Input: part model. Units: mm. Frame: model coordinates. Face numbers are marked on the shaded views. A direction names the side the tool comes from. Round coordinates to 2 decimals unless told otherwise and drop trailing zeros. Order: outer loops, then holes, each group sorted by start corner. A loop starts at its lowest first (then second) coordinate and runs counter-clockwise, first axis right, second up.
Item 1: Cut plane C-C on x = 10.25. Output: boundary loops of the cut face in (y, z).
Item 2: Line query: L1, parallel to Y at x = -1.8, z = -0.05; L2, parallel to Y at x = 4, z = 0; L3, parallel to X at y = -0.45, z = 0.3. Output: solid intervals per line, ascending.
Item 3: Mould query, pull axis Y, two halves, no side actions, for the marked faces 5, 6 and 7. Classes: released by +Y, released by -Y, zero draft, split by the parting line, or undercut.
Item 4: Cut plane B-B on y = 0. Output: boundary loops of the cut face in (x, z).
Item 5: Cut plane D-D on x = 3. Output: boundary loops of the cut face in (y, z), then the cut area to 3 significant figures.
Item 6: Cut plane A-A on x = -1.8. Output: boundary loops of the cut face in (y, z), then the cut area to 3 significant figures.
Item 7: Reachability of the marked faces 1, 2, 3 and 4 from +Z, -Z, +X, -X, +Y, -Y: full face, straight path, thin tool, end or side. Return the list, or none.
```python
from build123d import *

# Parameters (mm, degrees)
CUT_EXTRUDE1_DEPTH      = 13.655828697
CUT_EXTRUDE1_DEPTH_BACK = 13.655828697
CUT_EXTRUDE2_DEPTH      = 13.597618823
CUT_EXTRUDE2_DEPTH_BACK = 13.597618823


with BuildPart() as part:
    # Sketch1 → Revolve1 (revolve)
    with BuildSketch(Plane.XY, mode=Mode.PRIVATE) as revolve1_sk:
        with BuildLine():
            Line((0, 0.7), (-1.203701126, 1.266660038))
            ThreePointArc((-1.203701126, 1.266660038), (-2.550060523, 1.182120642), (-3.2, 0))
            Line((-3.2, 0), (12.5, 0))
            Line((12.5, 0), (12.5, 0.7))
            Line((12.5, 0.7), (0, 0.7))
        make_face()
    revolve(revolve1_sk.sketch.rotate(Axis((0, 0, 0), (1, 0, 0)), 90), axis=Axis((0, 0, 0), (1, 0, 0)))

    # Sketch2 → Cut-Extrude1 (cut, two sides: drawn at the far end of the back side and taken through both)
    with BuildSketch(Plane(origin=(0, 0, 0), x_dir=(1, 0, 0), z_dir=(0, 1, 0)).offset(-CUT_EXTRUDE1_DEPTH_BACK)):
        with BuildLine():
            Line((-3.012435565, 0.7), (0, 0.7))
            Line((0, 0.7), (-1.203701126, 1.266660038))
            ThreePointArc((-1.203701126, 1.266660038), (-2.218547495, 1.335970806), (-3.012435565, 0.7))
        make_face()
        with BuildLine():
            Line((-3.012435565, -0.7), (0, -0.7))
            Line((0, -0.7), (-1.203701126, -1.266660038))
            ThreePointArc((-1.203701126, -1.266660038), (-2.218547495, -1.335970806), (-3.012435565, -0.7))
        make_face()
    extrude(amount=CUT_EXTRUDE1_DEPTH + CUT_EXTRUDE1_DEPTH_BACK, mode=Mode.SUBTRACT)

    # Sketch3 → Cut-Extrude2 (cut, two sides: drawn at the far end of the back side and taken through both)
    with BuildSketch(Plane.XY.offset(-CUT_EXTRUDE2_DEPTH_BACK)):
        with BuildLine():
            Line((-1.530011672, 0.645837675), (-0.32, 0.14))
            Line((-0.32, 0.14), (10, 0.14))
            Line((10, 0.14), (10, 0.7))
            Line((10, 0.7), (12.5, 0.7))
            Line((12.5, 0.7), (12.5, -0.14))
            Line((12.5, -0.14), (-0.32, -0.14))
            Line((-0.32, -0.14), (-1.530011672, -0.645837675))
            ThreePointArc((-1.530011672, -0.645837675), (-2.5, 0), (-1.530011672, 0.645837675))
        make_face()
    extrude(amount=CUT_EXTRUDE2_DEPTH + CUT_EXTRUDE2_DEPTH_BACK, mode=Mode.SUBTRACT)


solid = part.part
```
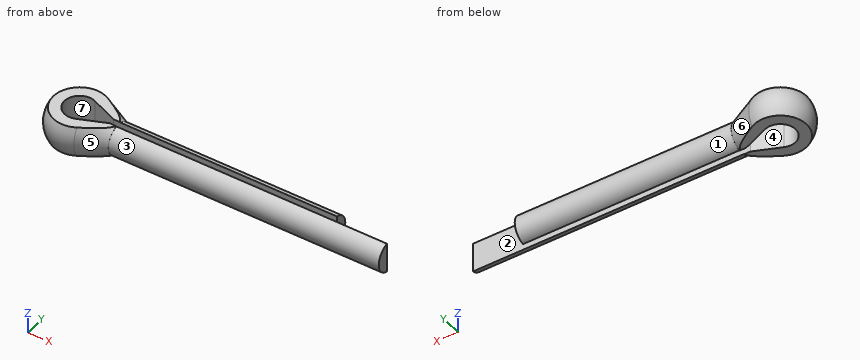
From the geometry:
1. outline: (-0.14, -0.69) - (-0.14, 0.69) arc R0.7 ccw to start
2. L1: y = -1.4 to -0.7, 0.7 to 1.4
2. L2: y = -0.7 to -0.14, 0.14 to 0.7
2. L3: x = -3.09 to -2.34, -1.06 to 12.5
3. face 5: released by -Y
3. face 6: released by +Y
3. face 7: undercut
4. outline: (-3.01, -0.7) - (-2.5, -0.7) - (-2.5, 0.7) - (-3.01, 0.7) arc R1.4 ccw to start
5. outline: (-0.14, -0.69) - (-0.14, 0.69) arc R0.7 ccw to start; (0.14, -0.69) arc R0.7 ccw to (0.14, 0.69) - close
5. area: 1.15 mm2
6. outline: (-1.21, -0.7) - (-0.7, -0.7) - (-0.7, 0.7) - (-1.21, 0.7) arc R1.4 ccw to start; (0.7, -0.7) - (1.21, -0.7) arc R1.4 ccw to (1.21, 0.7) - (0.7, 0.7) - close
6. area: 1.79 mm2
7. face 1: +X, +Y
7. face 2: +Z, -Z, +X
7. face 3: +X, -Y
7. face 4: +Z, -Z
